Geometry: final body of the model. Coordinates: model frame, mm. A direction names the side the tool comes from. Round coordinates to 2 decimals unless told otherwise and drop trailing zeros. Loops run counter-clockwise (first coordinate to the right, second up) from the corner with the lowest first, then second, coordinate; pieces in that order, holes last. Notation, with made-up numbers: M -14,16 L 45,16 A27 cw 45,53 Z; hole C 39.5,65.5 d6. An arc over 180 degrees is marked long. Answer as a JSON object with one key per item and string values.
Autodesk Inventor part; units mm, degrees
ref_plane "YZ Plane" through (0, 0, 0) normal (1, 0, 0) x (0, 1, 0)
ref_plane "XZ Plane" through (0, 0, 0) normal (0, 1, 0) x (-1, 0, 0)
ref_plane "XY Plane" through (0, 0, 0) normal (0, 0, 1) x (1, 0, 0)
sketch "スケッチ1" plane through (0, 0, 0) normal (0, 0, 1) x (1, 0, 0)
  circle A0 centre (0, 0) radius 2
  dimension "d0" = 4
extrude "押し出し1" add sketch "スケッチ1" along normal blind 12
sketch "スケッチ2" plane through (0, 0, 0) normal (0, 0, -1) x (-1, 0, 0)
  circle A0 centre (0, 0) radius 4
  dimension "d3" = 8
extrude "押し出し2" add sketch "スケッチ2" along normal blind 1.5
thread "ねじ1"
chamfer "面取り1" distance 0.5 angle 30 1 edges at (4, 0, -1.5) measured on face at (-0.7574, 1.0973, -1.5)
properties part number "ネジローヘッドm4,12" material "鋼、高強度、低合金"
1) First-contact query: pin 1 (4 mm diameter, centred on x = -2, z = 1.5, fed in from -Y); pin 2 (3 mm diameter, centred on x = 2.5, z = 7.5, fed in from -Y); pin 3 (2 mm diameter, centred on x = 0, z = 2, fed in from -Y). Flat tips, straight axial feed; report the tip coordinate or a pass-through.
Geometry results:
{"pin 1": "y = -3.94", "pin 2": "y = -1.73", "pin 3": "y = -2"}
2) Set-up query: faces 1 (the face through (0, 0, -1.5)), 2 (the face through (0, 2, 6)). Return all of +Z, -Z, +X, -X, +Y, -Y with unobstructed straight access to the full face (end or side cutting, diameter ignored); none if empty.
Geometry results:
{"face 1": "-Z, +X, -X, +Y, -Y", "face 2": "+Z"}
3) Cut plane D-D on z = -0.25. Return the cut outline in (x, y), and give its area (3 significant figures).
Geometry results:
{"outline": "C 0,0 d8", "area": "50.3 mm2"}
4) Cut plane C-C on z = 7.5. Return the cut outline in (x, y), and give its area (3 significant figures).
Geometry results:
{"outline": "C 0,0 d4", "area": "12.6 mm2"}
5) Cut plane A-A on y = 0. Return the cut outline in (x, z).
Geometry results:
{"outline": "M -4,-1.21 L -3.5,-1.5 L 3.5,-1.5 L 4,-1.21 L 4,0 L 2,0 L 2,12 L -2,12 L -2,0 L -4,0 Z"}
6) Line query: probe 1 along Z at (x, y) = (-1.5, 3); probe 2 along X at (y, z) = (0.5, 2.75). Output: solid intervals per line, ascending.
Geometry results:
{"probe 1": "-1.5 to 0", "probe 2": "-1.94 to 1.94"}
